The listing builds one solid part. Answer for the finished solid, in the listing's coordinates (mm). A direction names the side the tool comes from. Coordinates: 2 decimals unless noted, no trailing zeros. Loops run counter-clockwise (first coordinate to the right, second up) from the corner with the lowest first, then second, coordinate; pieces in that order, holes last. Notation, with made-up numbers: (-0.5, -19.5) -> (40.5, -19.5) arc R7 ccw to (40.5, -10.5) -> close; hole circle Ø11 at (35.5, -34). An arc over 180 degrees is marked (long way). Answer in a Markdown table with one row per item.
```python
from build123d import *

# Parameters (mm, degrees)
F1_DEPTH = 60
F3_DEPTH = 60
F4_R     = 5


with BuildPart() as f1:
    # F0 (on Front) → F1 (new body)
    with BuildSketch(Plane.XZ):
        Polygon((-100, -30), (100, -30), (100, 30), (40, 30), (40, -10), (-40, -10), (-40, 30), (-100, 30), align=None)
    extrude(amount=F1_DEPTH)

    # F2 (on face) → F3 (cut)
    with BuildSketch(Plane.YZ.offset(100)):
        with BuildLine():
            ThreePointArc((-20, 10), (-22.928932, 17.071068), (-30, 20))
            ThreePointArc((-30, 20), (-37.071068, 2.928932), (-20, 10))
        make_face()
    extrude(amount=-F3_DEPTH, mode=Mode.SUBTRACT)

    # F4
    f4_edges = [f1.edges().sort_by_distance(p)[0] for p in [
        (70, -60, 30),
        (70, 0, 30),
        (100, -30, 30),
        (-70, -60, 30),
        (-70, 0, 30),
        (-100, -30, 30),
        (100, 0, 0),
        (100, -60, 0),
        (-100, 0, 0),
        (-100, -60, 0),
    ]]
    fillet(f4_edges, radius=F4_R)


solid = f1.part
```
Item 1: A cutting plane is placed at B-B, the plane y = -38. Determine the outline of the cut face in (x, z).
Findings below:
| item | result |
|---|---|
| outline | (-100, -30) -> (100, -30) -> (100, 4) -> (40, 4) -> (40, -10) -> (-40, -10) -> (-40, 30) -> (-95, 30) arc R5 ccw to (-100, 25) -> close; (40, 16) -> (100, 16) -> (100, 25) arc R5 ccw to (95, 30) -> (40, 30) -> close |
Item 2: A cutting plane is placed at C-C, the plane y = -46.5. Determine the outline of the cut face in (x, z), plus the area to 3 significant figures.
Findings below:
| item | result |
|---|---|
| outline | (-100, -30) -> (100, -30) -> (100, 25) arc R5 ccw to (95, 30) -> (40, 30) -> (40, -10) -> (-40, -10) -> (-40, 30) -> (-95, 30) arc R5 ccw to (-100, 25) -> close |
| area | 8,790 mm2 |
Item 3: A cutting plane is placed at D-D, the plane x = 6.5. Determine the outline of the cut face in (y, z), plus the area to 3 significant figures.
Findings below:
| item | result |
|---|---|
| outline | (-60, -30) -> (0, -30) -> (0, -10) -> (-60, -10) -> close |
| area | 1,200 mm2 |
Item 4: Flat-ended cylindrical pins translate along their axes: pin 1 Ø1 at (y, z) = (-34, 6) entering from +X; pin 2 Ø20 at (y, z) = (-30, 6) entering from +X; pin 3 Ø18 at (x, y) = (-7.5, -33.5) entering from +Z. Find the tip coordinate at first contact, or state that the pin passes through.
Findings below:
| item | result |
|---|---|
| pin 1 | stops at x = -40 |
| pin 2 | stops at x = 100 |
| pin 3 | stops at z = -10 |
Item 5: Find the intervals of material crossed by probe 1 along Z at (x, y) = (82, -30); probe 2 along X at (y, z) = (-53, 25.5); probe 3 along Y at (x, z) = (84, 10), in increasing order.
Findings below:
| item | result |
|---|---|
| probe 1 | z = -30 to 0, 20 to 30 |
| probe 2 | x = -99.97 to -40, 40 to 99.97 |
| probe 3 | y = -60 to -40, -20 to 0 |
Item 6: A tool of negligible diameter and unlimited length cuts with its end or side. For faces 1 (the face through (1, -30, -10)), 2 (the face through (-68, -1, 28)), from which of +Z, -Z, +X, -X, +Y, -Y can it reach the whole face along a straight path? Write none if from no direction.
Findings below:
| item | result |
|---|---|
| face 1 | +Z, +Y, -Y |
| face 2 | +Z, +X, -X, +Y |
Item 7: A cutting plane is placed at A-A, the plane x = 44. Determine the outline of the cut face in (y, z).
Findings below:
| item | result |
|---|---|
| outline | (-60, -30) -> (0, -30) -> (0, 25) arc R5 ccw to (-5, 30) -> (-55, 30) arc R5 ccw to (-60, 25) -> close; hole circle Ø20 at (-30, 10) |
